The listing builds one solid part. Answer for the finished solid, in the listing's coordinates (mm). A direction names the side the tool comes from. Round coordinates to 2 decimals unless told otherwise and drop trailing zeros. Order: outer loops, then holes, each group sorted by start corner. A loop starts at its lowest first (then second) coordinate and runs counter-clockwise, first axis right, second up. Notation, with made-up numbers: (-14.5, -23) - (-0.5, -23) arc R32 cw to (-0.5, 3) - close; hole circle Ø3 at (-28, 16). An arc over 180 degrees is marked (long way). Use CSV: the item, a comma, the result in double quotes. Start each with the question number.
Item 1: Straight lines are drawn through the part: line 1 along Y through (x, z) = (35, 1.75); line 2 along X through (y, z) = (20.5, 3.3); line 3 along Y through (x, z) = (35.5, 1.7). For each, find the intervals that lie inside material, in ascending order. Write a range as [from, to].
Item 2: Find section D-D, the plane y = 10.5. Give the vertices of the cut face in (x, z), plus the area to 3 significant figures.
Item 3: Find section C-C, the plane x = 35. Give the vertices of the cut face in (y, z).
Item 4: A flat-ended cylindrical pin translates along its axis: P1, Ø2.5, axis at x = 14, y = 24, coming from the +Z side. Find the tip coordinate at first contact, or state that the pin passes through.
Item 5: Determine the mould class of faces 1 (the cylindrical face through (0.285, 47.699, 2.028)), 2 (the cylindrical face through (12.89, 25.01, 2.03)), 3 (the flat face through (20, 30, 0)), 4 (the flat face through (20, 0, 2)) for opening direction Y: +Y half, -Y half, draft (parallel to the pull), parting line (faces both ways), or undercut.
Item 6: For faces 5 (the flat face through (40, 24, 2)), 6 (the flat face through (27.06, 37.87, 1.97)), determine the directions among +Z, -Z, +X, -X, +Y, -Y from which every point of the face is accessible in a straight line to the end or side of a thin tool.
Item 7: Find section B-B, the plane x = 22. Give the vertices of the cut face in (y, z), plus the area to 3 significant figures.
Item 8: Find section A-A, the plane y = 3. Give the vertices of the cut face in (x, z), plus the area to 3 significant figures.
```python
from build123d import *

# Parameters (mm, degrees)
SKETCH_1_W          = 40
SKETCH_1_H          = 48
SKETCH_1_R          = 1.6
SKETCH_1_R_2        = 6
EXTRUDE_1_DEPTH     = 4
SKETCH_3_R          = 1.5
CUT_EXTRUDE_1_DEPTH = 63.60990337
CUT_EXTRUDE_2_DEPTH = 10
FILLET_1_R          = 1


with BuildPart() as part:
    # ｽｹｯﾁ1 → ﾎﾞｽ - 押し出し1 (new body)
    with BuildSketch(Plane.XY):
        with Locations((20, 24)):
            Rectangle(SKETCH_1_W, SKETCH_1_H)
        with Locations((5, 45)):
            Circle(SKETCH_1_R, mode=Mode.SUBTRACT)
        with Locations((5, 3)):
            Circle(SKETCH_1_R, mode=Mode.SUBTRACT)
        with Locations((35, 45)):
            Circle(SKETCH_1_R, mode=Mode.SUBTRACT)
        with Locations((35, 3)):
            Circle(SKETCH_1_R, mode=Mode.SUBTRACT)
        with Locations((22, 24)):
            Circle(SKETCH_1_R_2, mode=Mode.SUBTRACT)
    extrude(amount=EXTRUDE_1_DEPTH)

    # ｽｹｯﾁ3 → ｶｯﾄ - 押し出し1 (cut, through all)
    with BuildSketch(Plane.XY.offset(4)):
        with Locations((14, 24)):
            Circle(SKETCH_3_R)
    extrude(amount=-CUT_EXTRUDE_1_DEPTH, mode=Mode.SUBTRACT)

    # ｽｹｯﾁ4 → ｶｯﾄ - 押し出し2 (cut)
    with BuildSketch(Plane(origin=(0, 0, 0), x_dir=(-1, 0, 0), z_dir=(0, 0, -1))):
        with BuildLine():
            Line((-29.61454599, 42), (-25.019618207, 34.57742435))
            ThreePointArc((-25.019618207, 34.57742435), (-21.306285158, 34.978103649), (-17.672926458, 34.113181229))
            Line((-17.672926458, 34.113181229), (-11.288358882, 42))
            Line((-11.288358882, 42), (-29.61454599, 42))
        make_face()
        with BuildLine():
            ThreePointArc((-11, 24), (-11.514391519, 20.675542933), (-13.009457234, 17.662008143))
            Line((-13.009457234, 17.662008143), (-8, 11.473855089))
            Line((-8, 11.473855089), (-8, 36.526144911))
            Line((-8, 36.526144911), (-13.009457234, 30.337991857))
            ThreePointArc((-13.009457234, 30.337991857), (-11.514391519, 27.324457067), (-11, 24))
        make_face()
        with BuildLine():
            ThreePointArc((-17.672926458, 13.886818771), (-21.306285158, 13.021896351), (-25.019618207, 13.42257565))
            Line((-25.019618207, 13.42257565), (-29.61454599, 6))
            Line((-29.61454599, 6), (-11.288358882, 6))
            Line((-11.288358882, 6), (-17.672926458, 13.886818771))
        make_face()
    extrude(amount=-CUT_EXTRUDE_2_DEPTH, mode=Mode.SUBTRACT)

    # ﾌｨﾚｯﾄ1
    fillet_1_edges = [part.edges().sort_by_distance(p)[0] for p in [
        (13.009457234, 17.662008143, 2),
        (13.009457234, 30.337991857, 2),
        (8, 36.526144911, 2),
        (8, 11.473855089, 2),
        (25.019618207, 13.42257565, 2),
        (17.672926458, 13.886818771, 2),
        (11.288358882, 6, 2),
        (29.61454599, 6, 2),
        (17.672926458, 34.113181229, 2),
        (25.019618207, 34.57742435, 2),
        (29.61454599, 42, 2),
        (11.288358882, 42, 2),
        (0, 48, 2),
        (40, 48, 2),
        (40, 0, 2),
        (0, 0, 2),
    ]]
    fillet(fillet_1_edges, radius=FILLET_1_R)


solid = part.part
```
Worked out:
1,line 1,"y = [0, 1.4], [4.6, 43.4], [46.6, 48]"
1,line 2,"x = [0, 8], [11.57, 17.13], [26.87, 40]"
1,line 3,"y = [0, 1.48], [4.52, 43.48], [46.52, 48]"
2,outline,"(0, 0) - (14.93, 0) - (14.93, 4) - (0, 4) - close; (26.83, 0) - (40, 0) - (40, 4) - (26.83, 4) - close"
2,area,"112 mm²"
3,outline,"(0, 0) - (1.4, 0) - (1.4, 4) - (0, 4) - close; (4.6, 0) - (43.4, 0) - (43.4, 4) - (4.6, 4) - close; (46.6, 0) - (48, 0) - (48, 4) - (46.6, 4) - close"
4,P1,"passes through"
5,face 1,"+Y half"
5,face 2,"undercut"
5,face 3,"draft"
5,face 4,"-Y half"
6,face 5,"+Z, -Z, +X, +Y, -Y"
6,face 6,"+Z, -Z"
7,outline,"(0, 0) - (6, 0) - (6, 4) - (0, 4) - close; (13, 0) - (18, 0) - (18, 4) - (13, 4) - close; (30, 0) - (35, 0) - (35, 4) - (30, 4) - close; (42, 0) - (48, 0) - (48, 4) - (42, 4) - close"
7,area,"88.0 mm²"
8,outline,"(0, 0) - (3.4, 0) - (3.4, 4) - (0, 4) - close; (6.6, 0) - (33.4, 0) - (33.4, 4) - (6.6, 4) - close; (36.6, 0) - (40, 0) - (40, 4) - (36.6, 4) - close"
8,area,"134 mm²"
